The model under review builds one solid part; all positions refer to its coordinate system, in mm. Round coordinates to 2 decimals unless told otherwise and drop trailing zeros. Loops run counter-clockwise (first coordinate to the right, second up) from the corner with the lowest first, then second, coordinate; pieces in that order, holes last. Notation, with made-up numbers: M 47,73 L 77,73 A16 cw 77,85 Z; hole C 20.25,81 d11. An arc over 180 degrees is marked long. One line per question, with ' | ' between items.
from build123d import *

# Parameters (mm, degrees)
F0_W          = 26
F0_H          = 50
F1_DEPTH      = 5
F1_DEPTH_BACK = 5
F2_R          = 2
F3_DEPTH      = 26.001
F4_DEPTH      = 26.001


with BuildPart() as f1:
    # F0 (on Top) → F1 (new body, two sides)
    with BuildSketch(Plane.XY) as f1_sk:
        Rectangle(F0_W, F0_H)
    extrude(amount=F1_DEPTH)
    extrude(f1_sk.sketch, amount=-F1_DEPTH_BACK)

    # F2 (on face) → F3 (cut, through all)
    with BuildSketch(Plane(origin=(-13, 0, 0), x_dir=(0, -1, 0), z_dir=(-1, 0, 0))):
        Circle(F2_R)
        with Locations((20, 0)):
            Circle(F2_R)
        with Locations((-20, 0)):
            Circle(F2_R)
    extrude(amount=-F3_DEPTH, mode=Mode.SUBTRACT)

    # F2 (on face) → F4 (cut, through all)
    with BuildSketch(Plane(origin=(-13, 0, 0), x_dir=(0, -1, 0), z_dir=(-1, 0, 0))):
        Circle(F2_R)
        with Locations((20, 0)):
            Circle(F2_R)
        with Locations((-20, 0)):
            Circle(F2_R)
    extrude(amount=-F4_DEPTH, mode=Mode.SUBTRACT)


solid = f1.part
1) Add section B-B on y = 20. State the section outline as (x, z) points.
Output values:
outline: M -13,-5 L 13,-5 L 13,-2 L -13,-2 Z; M -13,2 L 13,2 L 13,5 L -13,5 Z
2) Insertion check: P1, Ø2.5, axis at y = 20, z = 0, coming from the +X side. The pin has a flat end and moves straight along its axis. Give the tip position at first contact, or say it passes through.
Output values:
P1: passes through
3) Add section C-C on x = -9.5. State the section outline as (y, z) points, then the cut area to 3 significant figures.
Output values:
outline: M -25,-5 L 25,-5 L 25,5 L -25,5 Z; hole C -20,0 d4; hole C 0,0 d4; hole C 20,0 d4 | area: 462 mm²
4) Add section A-A on z = 0. State the section outline as (x, y) points, then the cut area to 3 significant figures.
Output values:
outline: M -13,-25 L 13,-25 L 13,-22 L -13,-22 Z; M -13,-18 L 13,-18 L 13,-2 L -13,-2 Z; M -13,2 L 13,2 L 13,18 L -13,18 Z; M -13,22 L 13,22 L 13,25 L -13,25 Z | area: 988 mm²
5) For line 1 (Z direction, x = -2.75, y = 0); line 2 (Y direction, x = 1.75, z = -0.5); line 3 (Y direction, x = -11.5, z = -1.5), list the stretches that pass through material, from the lowest coordinate up.
Output values:
line 1: z = -5 to -2, 2 to 5 | line 2: y = -25 to -21.94, -18.06 to -1.94, 1.94 to 18.06, 21.94 to 25 | line 3: y = -25 to -21.32, -18.68 to -1.32, 1.32 to 18.68, 21.32 to 25
6) Add section D-D on y = -19. State the section outline as (x, z) points.
Output values:
outline: M -13,-5 L 13,-5 L 13,-1.73 L -13,-1.73 Z; M -13,1.73 L 13,1.73 L 13,5 L -13,5 Z
7) Mouldability with a two-part tool opening along Y and no side actions: class faces 1 (the flat face through (0, 0, 5)), 2 (the cylindrical face through (0, 0, -2)), 3 (the flat face through (0, 25, 0)) as +Y half, -Y half, draft (parallel to the pull), parting line (faces both ways), or undercut.
Output values:
face 1: draft | face 2: undercut | face 3: +Y half
